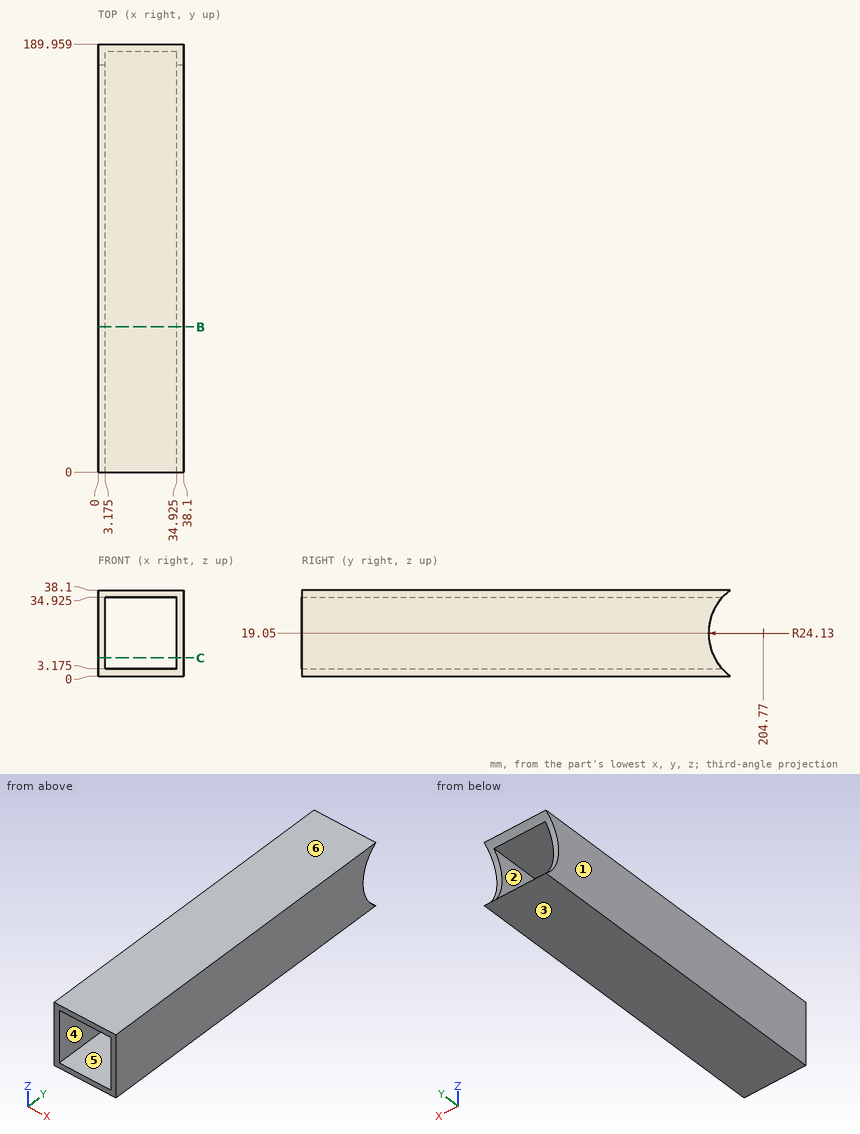
For this review, use the dimensioned drawing (mm, ordinates from the lowest corner) and the shaded views. A direction names the side the tool comes from. Round coordinates to 2 decimals unless told otherwise and drop trailing zeros. Loops run counter-clockwise (first coordinate to the right, second up) from the corner with the lowest first, then second, coordinate; pieces in that order, holes last. Notation, with made-up numbers: (-0.75, 0.5) -> (33.25, 0.5) arc R28 cw to (33.25, 39.5) -> close; hole circle Ø4 at (-32.75, 35.25). An arc over 180 degrees is marked (long way). Write item = value, one per line. Start each with the question number.
Item 1: For the marked faces 5 and 6, list the 3-axis set-ups (+Z, -Z, +X, -X, +Y, -Y) from which the entire face can be reached by the end or side of a thin tool; tool diameter is ignored.
Item 2: Mouldability with a two-part tool opening along Z and no side actions: class the marked faces 1, 2, 3 and 4 as released by +Z, released by -Z, zero draft, split by the parting line, or undercut.
Item 3: To check wall thickness, follow L1, parallel to X at y = 145.5, z = 31 (1 decimal). State the ranges of the line that lie inside material, in increasing order.
Item 4: Take a section at B-B on y = 64.5. Give the boundary of the cut face in (x, z) (1 decimal).
Item 5: Insertion check: pin 1 (8 mm diameter, centred on x = 9.5, z = 12.5, fed in from -Y); pin 2 (8 mm diameter, centred on x = 33, z = 24, fed in from +Y); pin 3 (8 mm diameter, centred on x = 16.5, z = 31.5, fed in from +Y) (1 decimal). Each pin has a flat end and moves straight along its axis. Give the tip position at first contact, or say it passes through.
Item 6: Take a section at C-C on z = 8. Give the boundary of the cut face in (x, y) (1 decimal).
Result:
q1.face_5 = +Y, -Y
q1.face_6 = +Z, +X, -X, +Y, -Y
q2.face_1 = zero draft
q2.face_2 = undercut
q2.face_3 = released by -Z
q2.face_4 = undercut
q3.L1 = 0 to 3.2, 34.9 to 38.1
q4.outline = (0, 0) -> (38.1, 0) -> (38.1, 38.1) -> (0, 38.1) -> close; hole (3.2, 3.2) -> (34.9, 3.2) -> (34.9, 34.9) -> (3.2, 34.9) -> close
q5.pin_1 = through
q5.pin_2 = 182.17
q5.pin_3 = 187.1
q6.outline = (0, 0) -> (3.2, 0) -> (3.2, 183.3) -> (0, 183.3) -> close; (34.9, 0) -> (38.1, 0) -> (38.1, 183.3) -> (34.9, 183.3) -> close
